```python
from build123d import *

# Parameters (mm, degrees)
F0_W     = 104
F0_H     = 46
F1_DEPTH = 34
F3_DEPTH = 46.001
F5_DEPTH = 46.0010001
F7_DEPTH = 68.0010001


with BuildPart() as f1:
    # F0 (on Front) → F1 (new body, symmetric)
    with BuildSketch(Plane.XZ):
        with Locations((4.4662589207, 23)):
            Rectangle(F0_W, F0_H)
    extrude(amount=F1_DEPTH, both=True)

    # F2 (on face) → F3 (cut, through all)
    with BuildSketch(Plane.XY.offset(46)):
        with BuildLine():
            Line((56.4662589207, 34), (36.4662589207, 34))
            add(Edge.make_bspline(
                [(36.4662589207, 34), (56.4662589207, 34), (56.4662589207, 15), (56.4662589207, 0)],
                knots=[0, 0, 0, 0, 39.4461658466, 39.4461658466, 39.4461658466, 39.4461658466], degree=3))
            Line((56.4662589207, 0), (56.4662589207, 34))
        make_face()
        with BuildLine():
            Line((56.4662589207, -34), (56.4662589207, 0))
            add(Edge.make_bspline(
                [(56.4662589207, 0), (56.4662589207, -15), (56.4662589207, -34), (36.4662589207, -34)],
                knots=[0, 0, 0, 0, 39.4461658466, 39.4461658466, 39.4461658466, 39.4461658466], degree=3))
            Line((36.4662589207, -34), (56.4662589207, -34))
        make_face()
    extrude(amount=-F3_DEPTH, mode=Mode.SUBTRACT)

    # F4 (on face) → F5 (cut, through all)
    with BuildSketch(Plane.XY.offset(46)):
        with BuildLine():
            Line((36.4662589207, 28), (-47.5337410793, 28))
            Line((-47.5337410793, 28), (-47.5337410793, -28))
            Line((-47.5337410793, -28), (36.4662589207, -28))
            add(Edge.make_bspline(
                [(49.7592477622, 0), (49.7592477622, -15), (49.7592477622, -28), (36.4662589207, -28)],
                knots=[0, 0, 0, 0, 30.9952182173, 30.9952182173, 30.9952182173, 30.9952182173], degree=3))
            add(Edge.make_bspline(
                [(36.4662589207, 28), (49.7518497669, 28), (49.7537801128, 15), (49.7592477622, 0)],
                knots=[0, 0, 0, 0, 30.9952182173, 30.9952182173, 30.9952182173, 30.9952182173], degree=3))
        make_face()
    extrude(amount=-F5_DEPTH, mode=Mode.SUBTRACT)

    # F6 (on face) → F7 (cut, through all)
    with BuildSketch(Plane.XZ.offset(34)):
        with BuildLine():
            Line((-47.5337410793, 0), (6.4662589207, 0))
            add(Edge.make_bspline(
                [(6.4662589207, 0), (-29.5337410793, 0), (-39.5337410793, 13), (-43.5337410793, 26.2024675506)],
                knots=[0, 0, 0, 0, 56.4497059845, 56.4497059845, 56.4497059845, 56.4497059845], degree=3))
            add(Edge.make_bspline(
                [(-43.5337410793, 26.2024675506), (-44.6908287704, 29.8478620036), (-46.2817139924, 35.2189317346), (-47.5337410793, 40)],
                knots=[0, 0, 0, 0, 14.3656500616, 14.3656500616, 14.3656500616, 14.3656500616], degree=3))
            Line((-47.5337410793, 40), (-47.5337410793, 0))
        make_face()
        with BuildLine():
            Line((-47.5337410793, 46), (-47.5337410793, 40))
            add(Edge.make_bspline(
                [(-47.5337410793, 40), (-47.5337410793, 42.4598008394), (-47.5337410793, 46), (-46.2817139924, 46)],
                knots=[0, 0, 0, 0, 6.1292390903, 6.1292390903, 6.1292390903, 6.1292390903], degree=3))
            Line((-46.2817139924, 46), (-47.5337410793, 46))
        make_face()
    extrude(amount=-F7_DEPTH, mode=Mode.SUBTRACT)


solid = f1.part
```
Build history of the part. All positions in model axes, mm. A direction names the side the tool comes from. Give positions to 0.01 mm unless a question says otherwise; leave off trailing zeros.
1) Probe line 1 along Y through (x, z) = (13.5, 44); line 2 along X through (y, z) = (3.5, 13); line 3 along Y through (x, z) = (38.5, 22.5). List the from-to ranges inside material, lowest first.
Values follow:
line 1: y = -34 to -28, 28 to 34
line 2: x = 49.75 to 56.46
line 3: y = -33.93 to -27.89, 27.89 to 33.93
2) Drop flat-ended pins along their axis: P1, Ø10, axis at y = 12.5, z = 22, coming from the +X side; P2, Ø3, axis at y = -20.5, z = 25, coming from the +X side; P3, Ø12, axis at y = 17, z = 39.5, coming from the +X side. Give the stop position or say it passes through.
Values follow:
P1: stops at x = 56.38
P2: stops at x = 55.06
P3: stops at x = 56.2
3) 3-axis set-ups, long thin cutter, end or side, ignore diameter. For faces 1 (the face through (-5, 28, 23)), 2 (the face through (-6, -34, 23)): which of +Z, -Z, +X, -X, +Y, -Y reach the whole face in a straight line?
Values follow:
face 1: +Z, -Z, -X
face 2: +Z, -Z, +X, -X, -Y
